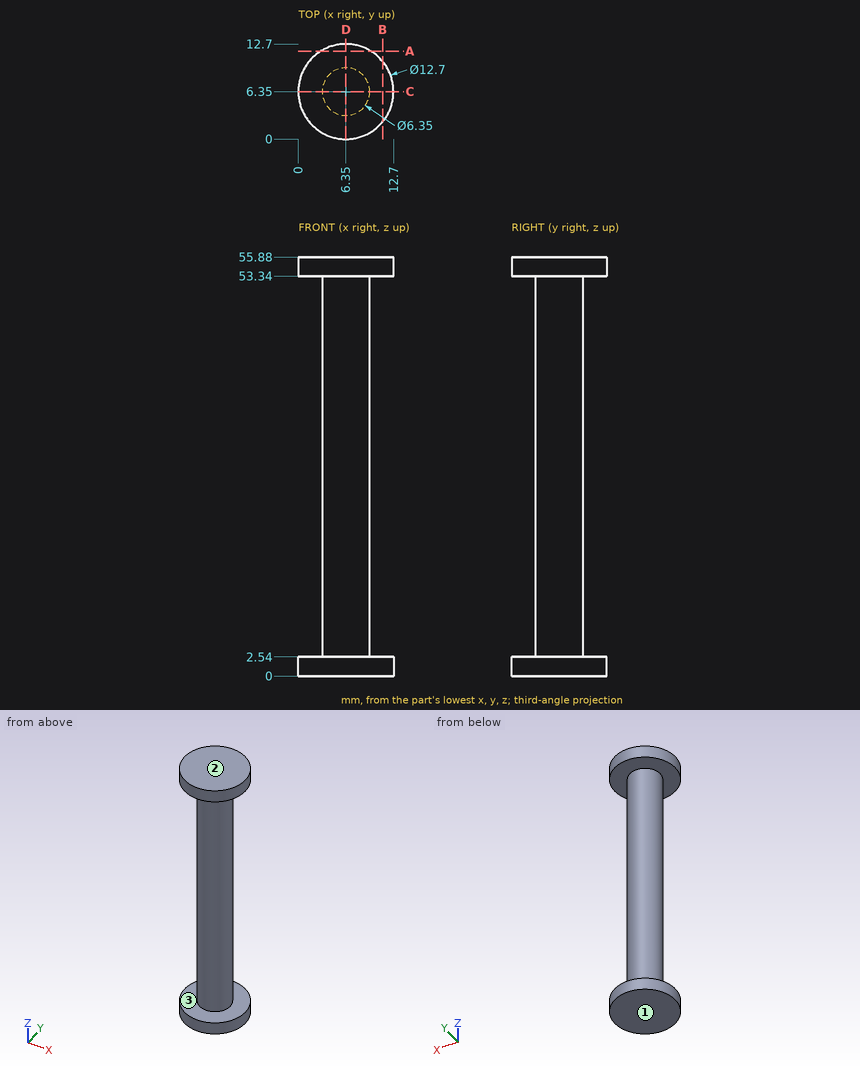
Design review of the part shown in the three views and the two pictorial views. Dimensions are in mm from the part's minimum x, y and z. Give positions to 0.01 mm unless a question says otherwise; leave off trailing zeros. Loops run counter-clockwise (first coordinate to the right, second up) from the corner with the lowest first, then second, coordinate; pieces in that order, holes last. Notation, with made-up numbers: (28, -39.75) -> (48, -39.75) arc R7 ccw to (48, -31.75) -> close; hole circle Ø9 at (-37.75, -23.75). An arc over 180 degrees is marked (long way). One line per question, with ' | ' between items.
1) We need section C-C (y = 6.35). Write out the cut boundary in (x, z) (3 decimals).
Resolved:
outline: (0, 0) -> (12.7, 0) -> (12.7, 2.54) -> (9.525, 2.54) -> (9.525, 53.34) -> (12.7, 53.34) -> (12.7, 55.88) -> (0, 55.88) -> (0, 53.34) -> (3.175, 53.34) -> (3.175, 2.54) -> (0, 2.54) -> close
2) The part is to be moulded in two halves that separate along Z. For the marked faces 1, 2 and 3, say which applies: +Z half, -Z half, draft (parallel to the pull), parting line (faces both ways), or undercut.
Resolved:
face 1: -Z half | face 2: +Z half | face 3: undercut
3) We need section B-B (x = 11.25). Write out the cut boundary in (y, z), plus the area to 3 significant figures.
Resolved:
outline: (2.31, 0) -> (10.39, 0) -> (10.39, 2.54) -> (2.31, 2.54) -> close; (2.31, 53.34) -> (10.39, 53.34) -> (10.39, 55.88) -> (2.31, 55.88) -> close | area: 41.0 mm2
4) Insertion check: pin 1 Ø1.5 at (x, z) = (4, 14) entering from +Y; pin 2 Ø2 at (y, z) = (5.5, 21) entering from -X (3 decimals); pin 3 Ø1 at (y, z) = (4, 47) entering from +X. Each pin has a flat end and moves straight along its axis. Give the tip position at first contact, or say it passes through.
Resolved:
pin 1: stops at y = 9.09 | pin 2: stops at x = 3.175 | pin 3: stops at x = 8.93
5) To check wall thickness, follow probe 1 along Z at (x, y) = (8.75, 2); probe 2 along Y at (x, z) = (6.5, 15); probe 3 along X at (y, z) = (9.25, 43.5). State the ranges of each line that lie inside material, in increasing order.
Resolved:
probe 1: z = 0 to 2.54, 53.34 to 55.88 | probe 2: y = 3.18 to 9.52 | probe 3: x = 5.06 to 7.64
6) We need section A-A (y = 11.75). Write out the cut boundary in (x, z).
Resolved:
outline: (3.01, 0) -> (9.69, 0) -> (9.69, 2.54) -> (3.01, 2.54) -> close; (3.01, 53.34) -> (9.69, 53.34) -> (9.69, 55.88) -> (3.01, 55.88) -> close
